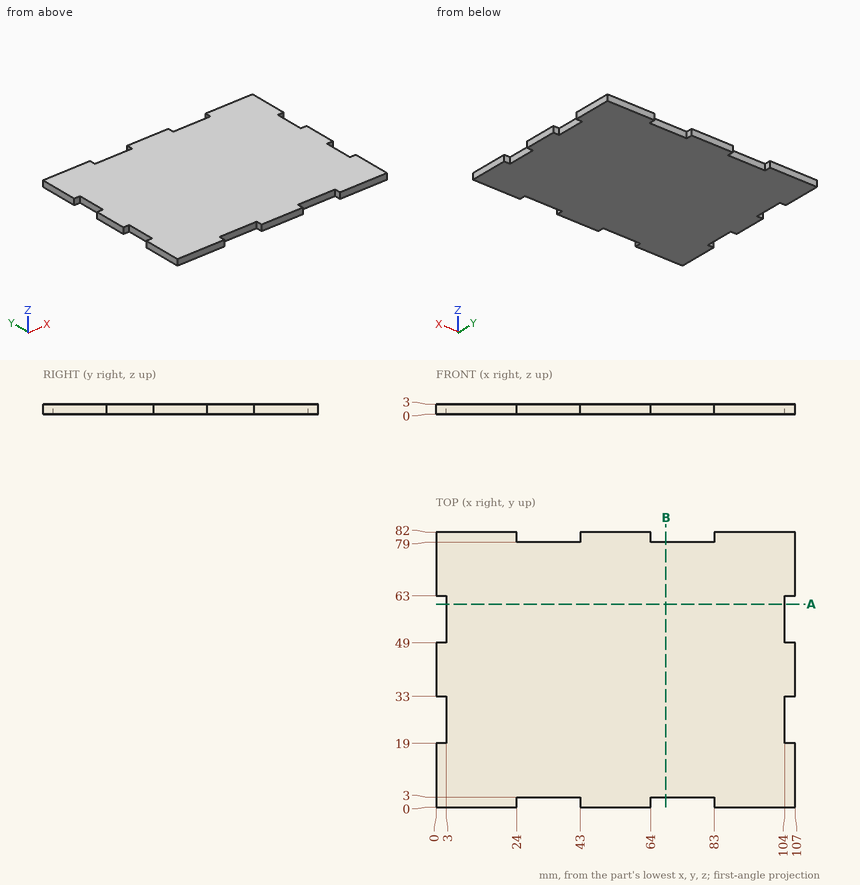
Geometry check sheet. Reference: drawing and pictorial views, mm from the part's lowest x, y, z. Coordinates: 2 decimals unless noted, no trailing zeros. Write each loop counter-clockwise with the first axis right and the second up, starting at its lowest first coordinate (ties: lowest second). Pieces come first, ordered by that corner, then holes.
Item 1: Cross-section at A-A on y = 60.5. Record the boundary of the cut face in (x, z), then the cut area to 3 significant figures.
Numbers:
outline: (3, 0) - (104, 0) - (104, 3) - (3, 3) - close
area: 303 mm2
Item 2: Depth check by flat-ended pin: pin 1 Ø0.9 at (x, z) = (106, 1.5) entering from -Y; pin 2 Ø1.5 at (y, z) = (58.5, 1.5) entering from -X; pin 3 Ø1.5 at (y, z) = (58, 1) entering from +X; pin 4 Ø1.5 at (x, z) = (34.5, 2) entering from -Y. Enter the tip coordinate at first touch or a pass-through.
Numbers:
pin 1: stops at y = 0
pin 2: stops at x = 3
pin 3: stops at x = 104
pin 4: stops at y = 3
Item 3: Cross-section at B-B on x = 68.5. Record the boundary of the cut face in (y, z), then the cut area to 3 significant figures.
Numbers:
outline: (3, 0) - (79, 0) - (79, 3) - (3, 3) - close
area: 228 mm2
Item 4: Scan lines: probe 1 along X at (y, z) = (62, 1.45); probe 2 along Y at (x, z) = (35, 1.95). Record each from-to range of solid material in increasing order.
Numbers:
probe 1: x = 3 to 104
probe 2: y = 3 to 79
